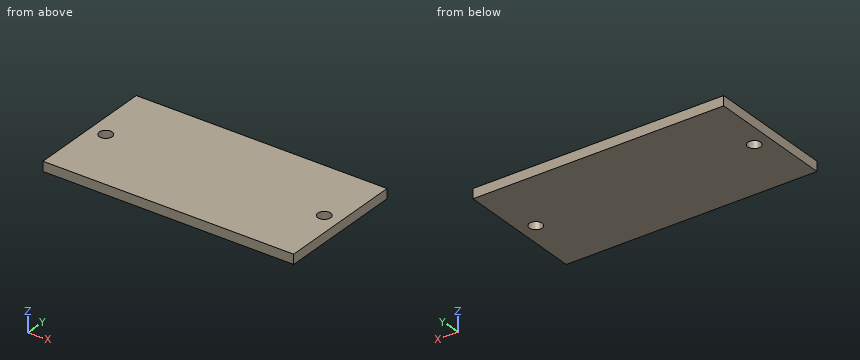
```python
from build123d import *

# Parameters (mm, degrees)
F0_W     = 39
F0_H     = 40
F0_R     = 2
F1_DEPTH = 3


with BuildPart() as f1:
    # F0 (on Top) → F1 (new body)
    with BuildSketch(Plane.XY):
        with Locations((-19.5, 20)):
            Rectangle(F0_W, F0_H)
        with Locations((-34, 20)):
            Circle(F0_R, mode=Mode.SUBTRACT)
        with Locations((19.5, 20)):
            Rectangle(F0_W, F0_H)
        with Locations((34, 20)):
            Circle(F0_R, mode=Mode.SUBTRACT)
    extrude(amount=F1_DEPTH)


solid = f1.part
```
For this review, take the finished solid that the model builds, in its own axes (mm). Round coordinates to 2 decimals unless told otherwise and drop trailing zeros. Loops run counter-clockwise (first coordinate to the right, second up) from the corner with the lowest first, then second, coordinate; pieces in that order, holes last.
(1) Wall thickness on line 1 along Y through (x, z) = (-34, 1.75); line 2 along X through (y, z) = (21, 0.3): over which ranges is each line inside the solid? List them lowest first.
Returned:
line 1: y = 0 to 18, 22 to 40
line 2: x = -39 to -35.73, -32.27 to 32.27, 35.73 to 39
(2) We need section B-B (x = 34). Give the boundary of the cut face in (y, z), plus the area to 3 significant figures.
Returned:
outline: (0, 0) - (18, 0) - (18, 3) - (0, 3) - close; (22, 0) - (40, 0) - (40, 3) - (22, 3) - close
area: 108 mm2
(3) We need section A-A (y = 20). Give the boundary of the cut face in (x, z), plus the area to 3 significant figures.
Returned:
outline: (-39, 0) - (-36, 0) - (-36, 3) - (-39, 3) - close; (-32, 0) - (32, 0) - (32, 3) - (-32, 3) - close; (36, 0) - (39, 0) - (39, 3) - (36, 3) - close
area: 210 mm2
